from build123d import *

# Parameters (mm, degrees)
PAD_DEPTH         = 20
PAD001_DEPTH      = 20
SKETCH002_R       = 15
POCKET_DEPTH      = 30.001
POCKET_DEPTH_BACK = -30.001
PAD002_DEPTH      = 5


with BuildPart() as part:
    # Sketch → Pad (new body, symmetric)
    with BuildSketch(Plane.XZ):
        with BuildLine():
            Line((20, 100), (-20, 100))
            Line((-20, 100), (-20, 60))
            Line((-20, 60), (-30, 40))
            Line((-30, 40), (-30, 0))
            Line((-30, 0), (-20, 0))
            Line((-20, 0), (-20, 30))
            ThreePointArc((20, 30), (0, 50), (-20, 30))
            Line((20, 30), (20, 0))
            Line((20, 0), (30, 0))
            Line((30, 0), (30, 40))
            Line((30, 40), (20, 60))
            Line((20, 60), (20, 100))
        make_face()
    extrude(amount=PAD_DEPTH, both=True)

    # Sketch001 → Pad001 (join, symmetric)
    with BuildSketch(Plane.YZ):
        with BuildLine():
            ThreePointArc((20, 100), (0, 120), (-20, 100))
            Line((-20, 100), (20, 100))
        make_face()
    extrude(amount=PAD001_DEPTH, both=True)

    # Sketch002 → Pocket (cut, two sides)
    with BuildSketch(Plane.YZ) as pocket_sk:
        with Locations((0, 100)):
            Circle(SKETCH002_R)
    extrude(amount=-POCKET_DEPTH, mode=Mode.SUBTRACT)
    extrude(pocket_sk.sketch, amount=-POCKET_DEPTH_BACK, mode=Mode.SUBTRACT)

    # Sketch003 → Pad002 (join, symmetric)
    with BuildSketch(Plane.XZ):
        Polygon((20, 60), (30, 60), (30, 40), align=None)
        Polygon((-30, 60), (-30, 40), (-20, 60), align=None)
    extrude(amount=PAD002_DEPTH, both=True)


solid = part.part
Verification items for the finished model (mm, model axes). A direction names the side the tool comes from. Give positions to 0.01 mm unless a question says otherwise; leave off trailing zeros. Write each loop counter-clockwise with the first axis right and the second up, starting at its lowest first coordinate (ties: lowest second). Pieces come first, ordered by that corner, then holes.
(1) Cross-section at A-A (y = 12). Enter the section's corners in (x, z), plus the area to 3 significant figures.
(2) Access from +Z, -Z, +X, -X, +Y, -Y to the whole of each face (thin tool, end or side, straight path). Record for faces 1 (the face through (-25, 12, 50)), 2 (the face through (26, 5, 52)), 3 (the face through (-25, -13, 50)).
(3) Gauge pin test, flat ends, axial feed: pin 1 (20 mm diameter, centred on y = -9.5, z = 75.5, fed in from +X); pin 2 (12 mm diameter, centred on y = -3.5, z = 105, fed in from -X); pin 3 (5 mm diameter, centred on x = -27, y = -0.5, fed in from +Z); pin 4 (8 mm diameter, centred on x = -23, y = 5.5, fed in from -Z). Record the tip position at first contact, or that the pin passes through.
(4) Cross-section at D-D (y = 0). Enter the section's corners in (x, z), plus the area to 3 significant figures.
(5) Cross-section at B-B (z = 8). Enter the section's corners in (x, y), plus the area to 3 significant figures.
(6) Cross-section at C-C (x = 21.5). Enter the section's corners in (y, z).
(7) Material ranges on line 1 (X direction, y = 11.5, z = 14.5); line 2 (Y direction, x = 3.5, z = 100); line 3 (X direction, y = -12, z = 60), recorded low to high.
(8) Mould release check, pull along Y, two halves, no side actions. Record for faces 4 (the face through (26, -5, 52)), 5 (the face through (0, 20, 62)), 6 (the face through (0.28, -3.252, 85.357)): +Y half, -Y half, draft (parallel to the pull), parting line (faces both ways), or undercut.
Worked out:
1. outline: (-30, 0) - (-20, 0) - (-20, 30) arc R20 cw to (20, 30) - (20, 0) - (30, 0) - (30, 40) - (20, 60) - (20, 91) - (-20, 91) - (-20, 60) - (-30, 40) - close; (-20, 109) - (20, 109) - (20, 116) - (-20, 116) - close
1. area: 3,090 mm2
2. face 1: +Z, -X, +Y
2. face 2: +Z, +X, +Y
2. face 3: +Z, -X, -Y
3. pin 1: stops at x = 20
3. pin 2: passes through
3. pin 3: stops at z = 60
3. pin 4: stops at z = 0
4. outline: (-30, 0) - (-20, 0) - (-20, 30) arc R20 cw to (20, 30) - (20, 0) - (30, 0) - (30, 60) - (20, 60) - (20, 85) - (-20, 85) - (-20, 60) - (-30, 60) - close; (-20, 115) - (20, 115) - (20, 120) - (-20, 120) - close
4. area: 2,970 mm2
5. outline: (-30, -20) - (-20, -20) - (-20, 20) - (-30, 20) - close; (20, -20) - (30, -20) - (30, 20) - (20, 20) - close
5. area: 800 mm2
6. outline: (-20, 0) - (20, 0) - (20, 57) - (5, 57) - (5, 60) - (-5, 60) - (-5, 57) - (-20, 57) - close
7. line 1: x = -30 to -20, 20 to 30
7. line 2: y = -20 to -15, 15 to 20
7. line 3: x = -20 to 20
8. face 4: -Y half
8. face 5: +Y half
8. face 6: undercut
